Check sheet for the modelled part. Datum: model origin and axes. Units: mm. A direction names the side the tool comes from. Coordinates: 2 decimals unless noted, no trailing zeros. Write each loop counter-clockwise with the first axis right and the second up, starting at its lowest first coordinate (ties: lowest second). Pieces come first, ordered by that corner, then holes. Notation, with made-up numbers: M 82,76 L 109,76 A21 cw 109,81 Z; hole C 19.25,-18.75 d1. An arc over 180 degrees is marked long. Answer as CSV lines item,"result".
from build123d import *

# Parameters (mm, degrees)
F0_W     = 30
F0_H     = 30
F0_W_2   = 24
F0_H_2   = 24
F1_DEPTH = 200
F2_R     = 1
F3_R     = 3
F5_DEPTH = 30.001


with BuildPart() as f1:
    # F0 (on Top) → F1 (new body)
    with BuildSketch(Plane.XY):
        Rectangle(F0_W, F0_H)
        Rectangle(F0_W_2, F0_H_2, mode=Mode.SUBTRACT)
    extrude(amount=F1_DEPTH)

    # F2
    f2_edges = [f1.edges().sort_by_distance(p)[0] for p in [
        (-12, -12, 100),
        (-12, 12, 100),
        (12, 12, 100),
        (12, -12, 100),
    ]]
    fillet(f2_edges, radius=F2_R)

    # F3
    f3_edges = [f1.edges().sort_by_distance(p)[0] for p in [
        (-15, 15, 100),
        (-15, -15, 100),
        (15, 15, 100),
        (15, -15, 100),
    ]]
    fillet(f3_edges, radius=F3_R)

    # F4 (on face) → F5 (cut, through all)
    with BuildSketch(Plane.XZ.offset(15)):
        Polygon((-12, 200), (-12, 197), (12, 173), (12, 200), align=None)
        Polygon((-12, 200), (-15, 200), (-12, 197), align=None)
        Polygon((12, 200), (12, 173), (15, 170), (15, 200), align=None)
    extrude(amount=-F5_DEPTH, mode=Mode.SUBTRACT)


solid = f1.part
1) Section check A-A, the plane x = 6.25. Record the boundary of the cut face in (y, z).
Answer key:
outline,"M -15,0 L -12,0 L -12,178.75 L -15,178.75 Z; M 12,0 L 15,0 L 15,178.75 L 12,178.75 Z"
2) Tool access check on faces 1 (the face through (-14, 0, 0)), 2 (the face through (0, 12, 97)). Record the directions out of +Z, -Z, +X, -X, +Y, -Y that give a thin tool (end or side, any length) a straight path to the whole face; none if there is none.
Answer key:
face 1,"-Z, +X, -X, +Y, -Y"
face 2,"+Z, -Z"
3) Thickness scan on line 1 along X through (y, z) = (5.5, 92); line 2 along Y through (x, z) = (11.25, 159); line 3 along X through (y, z) = (11.5, 116). Record the ranges inside material, lowest first.
Answer key:
line 1,"x = -15 to -12, 12 to 15"
line 2,"y = -15 to -11.97, 11.97 to 15"
line 3,"x = -15 to -11.87, 11.87 to 15"
4) Section check B-B, the plane z = 92.5. Record the boundary of the cut face in (x, y), plus the area to 3 significant figures.
Answer key:
outline,"M -15,-12 A3 ccw -12,-15 L 12,-15 A3 ccw 15,-12 L 15,12 A3 ccw 12,15 L -12,15 A3 ccw -15,12 Z; hole M -12,-11 A1 ccw -11,-12 L 11,-12 A1 ccw 12,-11 L 12,11 A1 ccw 11,12 L -11,12 A1 ccw -12,11 Z"
area,"317 mm2"
5) Mould release check, pull along Y, two halves, no side actions. Record for faces 3 (the face through (12, 0, 85)), 4 (the face through (0, 13, 185)), 5 (the face through (0, 15, 97)): pulls with the +Y half, pulls with the -Y half, needs draft (parallel to the pull), parting line crosses it, or undercut.
Answer key:
face 3,"undercut"
face 4,"needs draft"
face 5,"pulls with the +Y half"
6) Section check C-C, the plane y = -7.5. Record the boundary of the cut face in (x, z).
Answer key:
outline,"M -15,0 L -12,0 L -12,197 L -15,200 Z; M 12,0 L 15,0 L 15,170 L 12,173 Z"
